```python
from build123d import *

# Parameters (mm, degrees)
F1_DEPTH = 25


with BuildPart() as f1:
    # F0 (on Top) → F1 (new body)
    with BuildSketch(Plane.XY):
        with BuildLine():
            ThreePointArc((27.813243, 193.999363), (40.541165, 188.727285), (45.813243, 175.999363))
            Line((45.813243, 175.999363), (45.813243, 23.999363))
            ThreePointArc((45.813243, 23.999363), (40.541165, 11.271441), (27.813243, 5.999363))
            Line((27.813243, 5.999363), (-59.436757, 5.999363))
            Line((-59.436757, 5.999363), (-59.436757, -20.000637))
            Line((-59.436757, -20.000637), (166.563243, -20.000637))
            Line((166.563243, -20.000637), (166.563243, 5.999363))
            Line((166.563243, 5.999363), (79.313243, 5.999363))
            ThreePointArc((79.313243, 5.999363), (66.585321, 11.271441), (61.313243, 23.999363))
            Line((61.313243, 23.999363), (61.313243, 175.999363))
            ThreePointArc((61.313243, 175.999363), (66.585321, 188.727285), (79.313243, 193.999363))
            Line((79.313243, 193.999363), (166.563243, 193.999363))
            Line((166.563243, 193.999363), (166.563243, 219.999363))
            Line((166.563243, 219.999363), (-59.436757, 219.999363))
            Line((-59.436757, 219.999363), (-59.436757, 193.999363))
            Line((-59.436757, 193.999363), (27.813243, 193.999363))
        make_face()
    extrude(amount=F1_DEPTH)


solid = f1.part
```
Design review of the part built by this model. Coordinates are the model's own, in mm. A direction names the side the tool comes from. Coordinates: 2 decimals unless noted, no trailing zeros. Loops run counter-clockwise (first coordinate to the right, second up) from the corner with the lowest first, then second, coordinate; pieces in that order, holes last. Notation, with made-up numbers: M 23,69.5 L 82,69.5 A19 cw 82,87.5 Z; hole C 82,-8.5 d6. An arc over 180 degrees is marked long. One line per question, with ' | ' between items.
(1) We need section B-B (z = 4.25). Give the boundary of the cut face in (x, y), and give its area (3 significant figures).
Filled in:
outline: M -59.44,-20 L 166.56,-20 L 166.56,6 L 79.31,6 A18 cw 61.31,24 L 61.31,176 A18 cw 79.31,194 L 166.56,194 L 166.56,220 L -59.44,220 L -59.44,194 L 27.81,194 A18 cw 45.81,176 L 45.81,24 A18 cw 27.81,6 L -59.44,6 Z | area: 14,900 mm^2
(2) For pin 1 Ø12 at (y, z) = (21, 18) entering from -X; pin 2 Ø1 at (y, z) = (66, 13) entering from -X; pin 3 Ø1.5 at (y, z) = (80.5, 8.5) entering from +X, all flat-tipped, find the tip position at first contact; note any pin that passes through.
Filled in:
pin 1: stops at x = 43.4 | pin 2: stops at x = 45.81 | pin 3: stops at x = 61.31
(3) We need section A-A (x = 113). Give the boundary of the cut face in (y, z).
Filled in:
outline: M -20,0 L 6,0 L 6,25 L -20,25 Z; M 194,0 L 220,0 L 220,25 L 194,25 Z
(4) Draft analysis for pull direction Y (two halves, no side actions). For faces 4 (the face through (55, 219.999, 12)), 5 (the face through (61.313, 99, 12)), 6 (the face through (-59.437, 207, 12)), state which applies: released by +Y, released by -Y, zero draft, split by the parting line, or undercut.
Filled in:
face 4: released by +Y | face 5: undercut | face 6: zero draft
(5) We need section D-D (x = 32). Give the boundary of the cut face in (y, z).
Filled in:
outline: M -20,0 L 6.49,0 L 6.49,25 L -20,25 Z; M 193.51,0 L 220,0 L 220,25 L 193.51,25 Z
(6) Wall thickness on probe 1 along Y at (x, z) = (-25, 21); probe 2 along X at (y, z) = (37.5, 21.25); probe 3 along X at (y, z) = (189.5, 11.25): over which ranges is each line inside the solid? List them lowest first.
Filled in:
probe 1: y = -20 to 6, 194 to 220 | probe 2: x = 45.81 to 61.31 | probe 3: x = 39.72 to 67.41
(7) Machinability: for faces 1 (the face through (53, 92, 0)), 2 (the face through (40.68, 11.41, 12.32)), 3 (the face through (66.45, 188.59, 12.32)), which of the approach directions +Z, -Z, +X, -X, +Y, -Y give a long, thin tool a straight path to every point of the face, cutting with its end or side? Answer none if there is none.
Filled in:
face 1: -Z, +X, -X, +Y, -Y | face 2: +Z, -Z, -X | face 3: +Z, -Z, +X
(8) We need section C-C (y = 63). Give the boundary of the cut face in (x, z), and give its area (4 significant figures).
Filled in:
outline: M 45.81,0 L 61.31,0 L 61.31,25 L 45.81,25 Z | area: 387.5 mm^2
